Input: dimensioned drawing with shaded views. Units: mm. Origin: part minimum x, y, z. Round coordinates to 2 decimals unless told otherwise and drop trailing zeros. Order: outer loops, then holes, each group sorted by start corner. A loop starts at its lowest first (then second) coordinate and runs counter-clockwise, first axis right, second up.
Item 1: Line query: L1, parallel to Z at x = 7.25, y = 1.95; L2, parallel to X at y = 1.75, z = 15.75. Output: solid intervals per line, ascending.
Item 2: Cut plane B-B on y = 1.5. Output: boundary loops of the cut face in (x, z), then the cut area to 3 significant figures.
Item 3: Cut plane C-C on z = 6.25. Output: boundary loops of the cut face in (x, y), then the cut area to 3 significant figures.
Item 4: First-contact query: pin 1 (1 mm diameter, centred on x = 7.5, y = 1, fed in from -Z); pin 2 (0.6 mm diameter, centred on y = 1.5, z = 10, fed in from -X). Flat tips, straight axial feed; report the tip coordinate or a pass-through.
Item 5: Cut plane A-A on x = 2. Output: boundary loops of the cut face in (y, z).
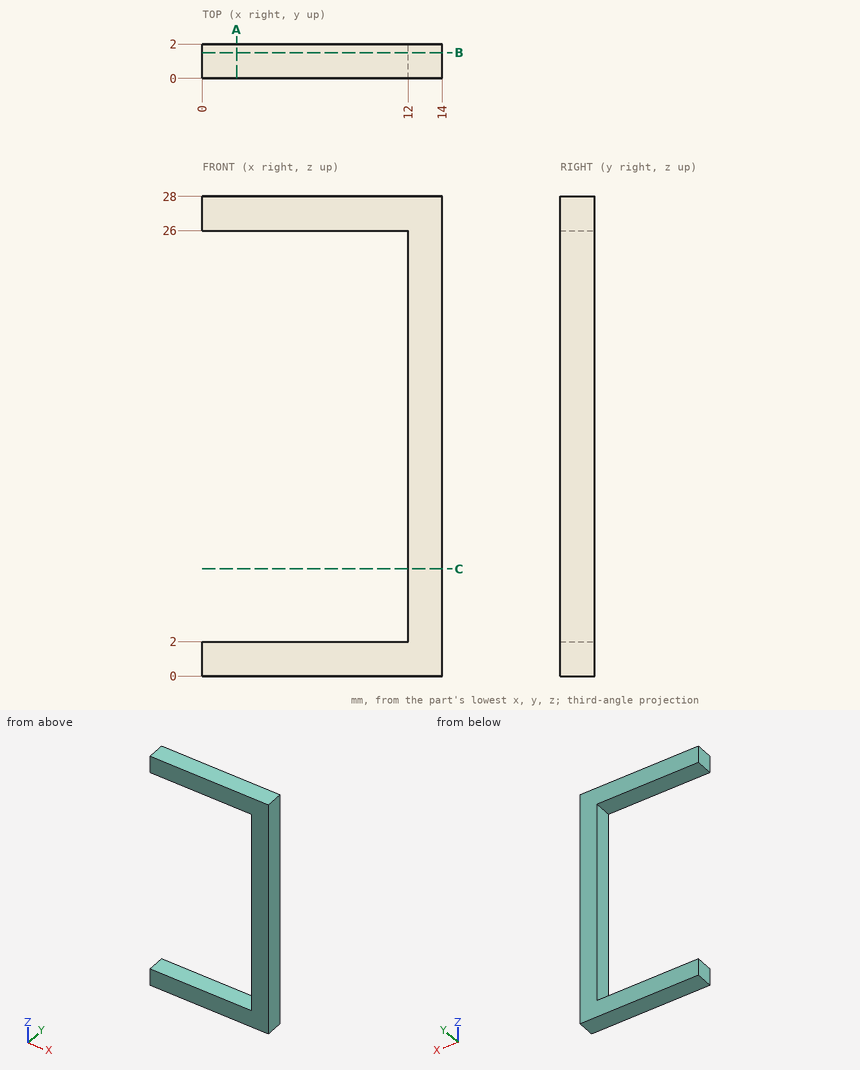
From the geometry:
1. L1: z = 0 to 2, 26 to 28
1. L2: x = 12 to 14
2. outline: (0, 0) - (14, 0) - (14, 28) - (0, 28) - (0, 26) - (12, 26) - (12, 2) - (0, 2) - close
2. area: 104 mm2
3. outline: (12, 0) - (14, 0) - (14, 2) - (12, 2) - close
3. area: 4.00 mm2
4. pin 1: stops at z = 0
4. pin 2: stops at x = 12
5. outline: (0, 0) - (2, 0) - (2, 2) - (0, 2) - close; (0, 26) - (2, 26) - (2, 28) - (0, 28) - close
